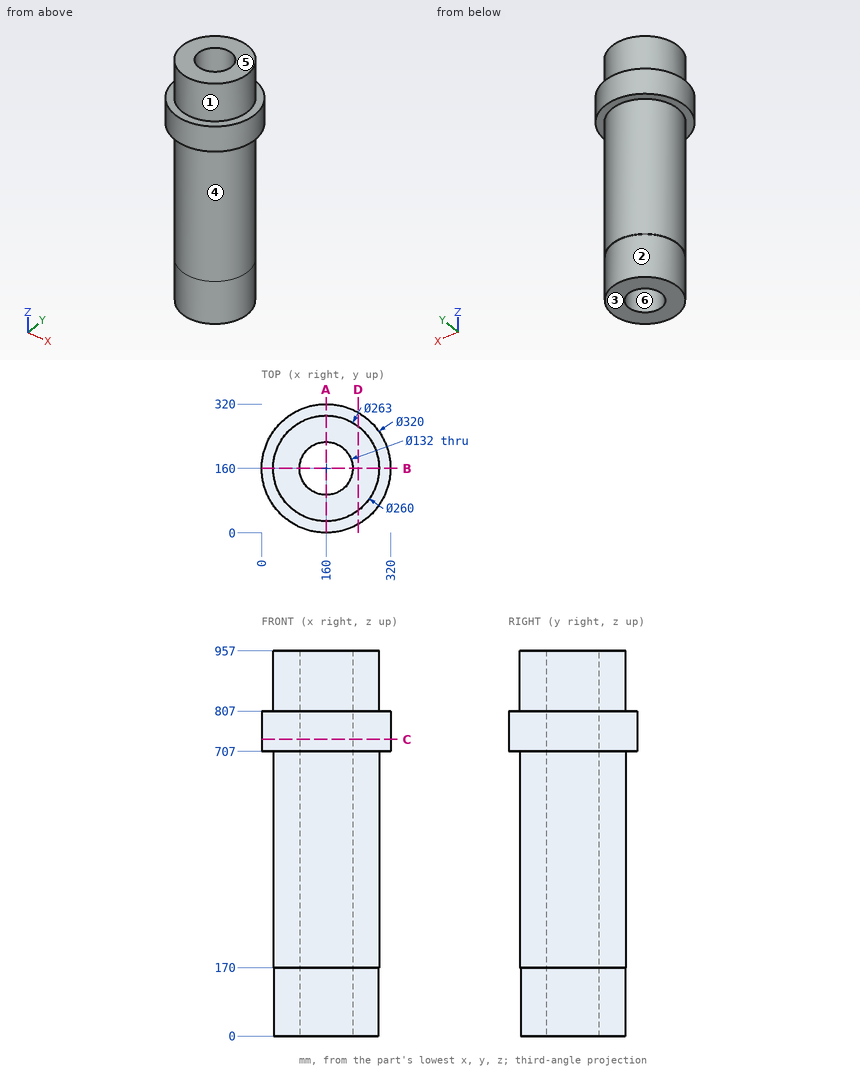
Verification items for this drawing (mm, ordinates from the low corner). A direction names the side the tool comes from. Coordinates: 2 decimals unless noted, no trailing zeros. Order: outer loops, then holes, each group sorted by start corner. A loop starts at its lowest first (then second) coordinate and runs counter-clockwise, first axis right, second up. Notation, with made-up numbers: (-33.75, 20) -> (5.25, 20) arc R27 ccw to (5.25, 56) -> close; hole circle Ø2 at (81, 61). An arc over 180 degrees is marked (long way). Answer as CSV lines item,"result". Start each with the question number.
1) Release check for a two-part mould opening along X. For the marked faces 4, 5 and 6 record: released by +X, released by -X, zero draft, split by the parting line, or undercut.
2) Cross-section at A-A, the plane x = 160. Record the boundary of the cut face in (y, z), then the cut area to 3 significant figures.
3) Cross-section at D-D, the plane x = 239.5. Record the boundary of the cut face in (y, z), then the cut area to 3 significant figures.
4) Set-up check for the marked faces 1, 2 and 3: record each of +Z, -Z, +X, -X, +Y, -Y from which the full face is reachable in a straight line by a thin tool's end or side.
5) Material ranges on L1, parallel to X at y = 160, z = 395; L2, parallel to Z at x = 277.5, y = 236; L3, parallel to X at y = 127.5, z = 553, recorded low to high. Write a range as [from, to].
6) Cross-section at C-C, the plane z = 737. Record the boundary of the cut face in (x, y).
7) Gauge pin test, flat ends, axial feed: pin 1 Ø10 at (x, z) = (171.5, 238) entering from -Y; pin 2 Ø8 at (y, z) = (49, 596) entering from -X; pin 3 Ø10 at (x, z) = (113, 698.5) entering from +Y. Record the tip position at first contact, or that the pin passes through.
Conclusion:
1,face 4,"split by the parting line"
1,face 5,"zero draft"
1,face 6,"undercut"
2,outline,"(0, 707) -> (28.5, 707) -> (28.5, 170) -> (30, 170) -> (30, 0) -> (94, 0) -> (94, 957) -> (28.5, 957) -> (28.5, 807) -> (0, 807) -> close; (226, 0) -> (290, 0) -> (290, 170) -> (291.5, 170) -> (291.5, 707) -> (320, 707) -> (320, 807) -> (291.5, 807) -> (291.5, 957) -> (226, 957) -> close"
2,area,"131,000 mm²"
3,outline,"(21.15, 707) -> (55.25, 707) -> (55.25, 170) -> (57.14, 170) -> (57.14, 0) -> (262.86, 0) -> (262.86, 170) -> (264.75, 170) -> (264.75, 707) -> (298.85, 707) -> (298.85, 807) -> (264.75, 807) -> (264.75, 957) -> (55.25, 957) -> (55.25, 807) -> (21.15, 807) -> close"
3,area,"207,000 mm²"
4,face 1,"+Z"
4,face 2,"-Z"
4,face 3,"-Z, +X, -X, +Y, -Y"
5,L1,"x = [28.5, 94], [226, 291.5]"
5,L2,"z = [707, 807]"
5,L3,"x = [32.58, 102.56], [217.44, 287.42]"
6,outline,"circle Ø320 at (160, 160); hole circle Ø132 at (160, 160)"
7,pin 1,"stops at y = 28.66"
7,pin 2,"stops at x = 83.56"
7,pin 3,"stops at y = 284.61"
